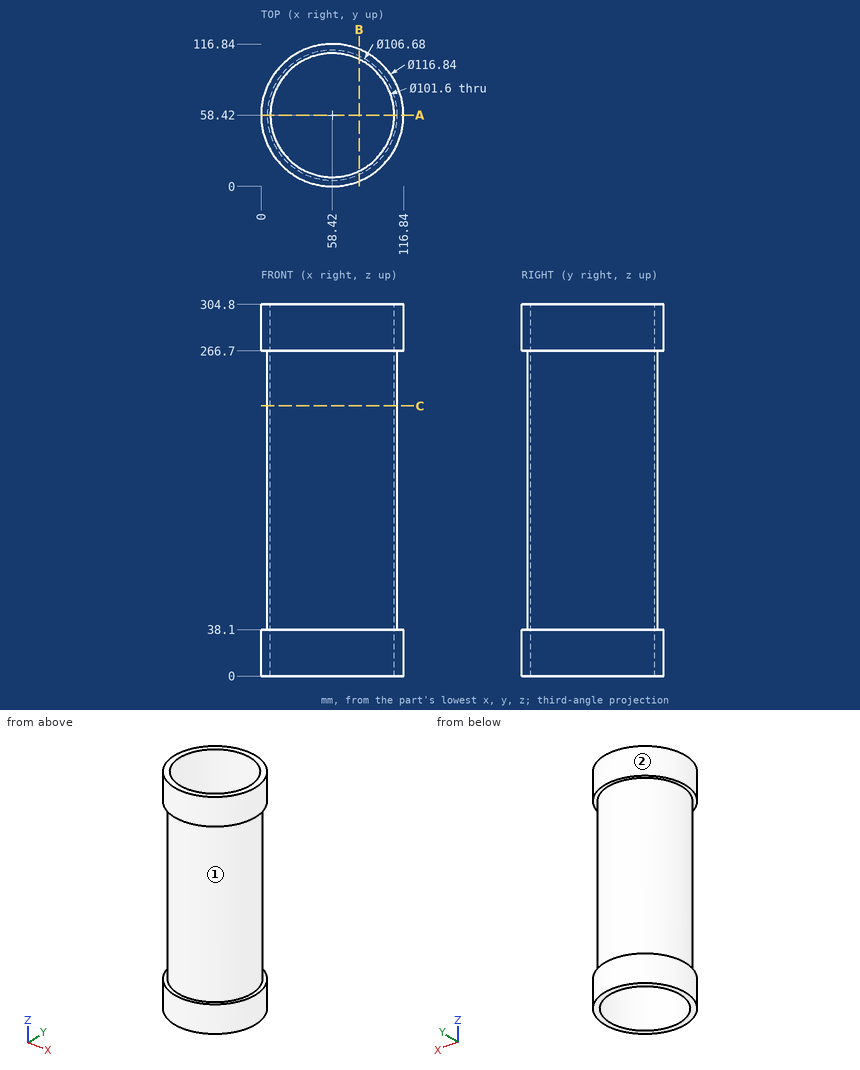
Can you work these out from the drawing? Everything is in mm from the part's minimum corner. Coordinates: 2 decimals unless noted, no trailing zeros. Loops run counter-clockwise (first coordinate to the right, second up) from the corner with the lowest first, then second, coordinate; pieces in that order, holes last. Notation, with made-up numbers: (69, 13.25) - (98, 13.25) arc R22 ccw to (98, 27.25) - close; hole circle Ø10 at (6.25, 17). An arc over 180 degrees is marked (long way). Put each result on its own line as item: value. Start each with the question number.
Item 1: Suppose I cut it at C-C (z = 221.5). Please give me the cut outline in (x, y), and give its area (3 significant figures).
Item 2: For pin 1 (8 mm diameter, centred on y = 43.5, z = 137.5, fed in from +X); pin 2 (6 mm diameter, centred on y = 101, z = 49, fed in from +X); pin 3 (1 mm diameter, centred on x = 64, z = 61, fed in from -Y), each with a flat end and sliding along its axis, tell me the tip position at first contact or that it passes through.
Item 3: Suppose I cut it at B-B (x = 80.5). Please give me the cut outline in (y, z).
Item 4: Suppose I cut it at A-A (y = 58.42). Please give me the cut outline in (x, z), and give its area (3 significant figures).
Item 5: If I drill on line 1 along Z through (x, y) = (84, 7); line 2 along X through (y, z) = (58, 120), over which ranges is the centre line in solid material (lowest first)?
Item 6: If we mould it in two halves opening along Z, with no side actions, what happens to the marked faces 1 and 2? For each: +Z half, -Z half, draft (parallel to the pull), parting line (faces both ways), or undercut.
Here are the results:
1. outline: circle Ø106.68 at (58.42, 58.42); hole circle Ø101.6 at (58.42, 58.42)
1. area: 831 mm²
2. pin 1: x = 110.63
2. pin 2: x = 94.18
2. pin 3: y = 5.32
3. outline: (4.33, 0) - (12.67, 0) - (12.67, 304.8) - (4.33, 304.8) - (4.33, 266.7) - (9.86, 266.7) - (9.86, 38.1) - (4.33, 38.1) - close; (104.17, 0) - (112.51, 0) - (112.51, 38.1) - (106.98, 38.1) - (106.98, 266.7) - (112.51, 266.7) - (112.51, 304.8) - (104.17, 304.8) - close
4. outline: (0, 0) - (7.62, 0) - (7.62, 304.8) - (0, 304.8) - (0, 266.7) - (5.08, 266.7) - (5.08, 38.1) - (0, 38.1) - close; (109.22, 0) - (116.84, 0) - (116.84, 38.1) - (111.76, 38.1) - (111.76, 266.7) - (116.84, 266.7) - (116.84, 304.8) - (109.22, 304.8) - close
4. area: 2,320 mm²
5. line 1: 0 to 38.1, 266.7 to 304.8
5. line 2: 5.08 to 7.62, 109.22 to 111.76
6. face 1: undercut
6. face 2: draft
